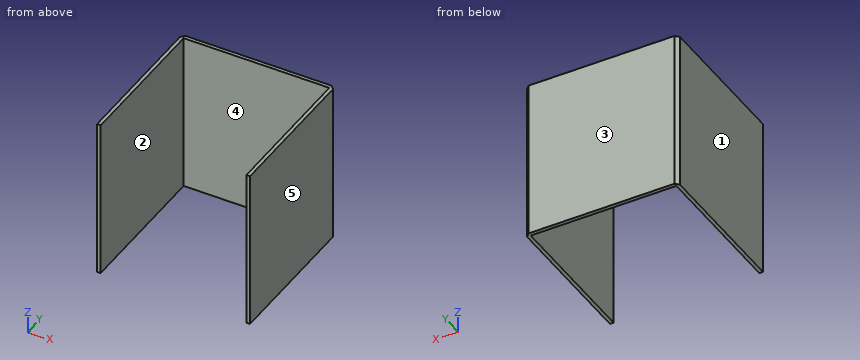
Autodesk Inventor part; units mm, degrees
ref_plane "YZ Plane" through (0, 0, 0) normal (1, 0, 0) x (0, 1, 0)
ref_plane "XZ Plane" through (0, 0, 0) normal (0, 1, 0) x (-1, 0, 0)
ref_plane "XY Plane" through (0, 0, 0) normal (0, 0, 1) x (1, 0, 0)
sketch "Sketch1" plane through (0, 0, 0) normal (0, 0, 1) x (1, 0, 0)
  line L0 (10, -10) -> (-10, -10)
  line L1 (-10, -10) -> (-10, 10)
  line L2 (-10, 10) -> (10, 10)
  line L3 (10, 10) -> (10, -10)
  line L4 (10, -10) -> (-10, 10) construction
  line L5 (-10, -10) -> (10, 10) construction
  line L6 (10.5, 10.5) -> (-10.5, 10.5)
  line L7 (-10.5, 10.5) -> (-10.5, -10.5)
  line L8 (-10.5, -10.5) -> (10.5, -10.5)
  line L9 (10.5, -10.5) -> (10.5, 10.5)
  line L10 (-10.5, -10) -> (10.5, -10)
  point P0 (0, 0)
  dimension "d0" = 20
  dimension "d1" = 20
  dimension "d2" = 0.5
extrude "Extrusion1" add sketch "Sketch1" along normal mid plane 22 contours L3 L2 L1 L10 L7 L6 L9
chamfer "Chamfer1" distance 0.5 angle 45 2 edges at (10.5, 10.5, 0) (-10.5, 10.5, 0)
properties part number "cover"
Can you work these out from the model? Positions are in its coordinate system, mm. Face numbers are marked on the shaded views. A direction names the side the tool comes from. Give positions to 0.01 mm unless a question says otherwise; leave off trailing zeros. Order: outer loops, then holes, each group sorted by start corner. A loop starts at its lowest first (then second) coordinate and runs counter-clockwise, first axis right, second up. Notation, with made-up numbers: M 34.25,84.5 L 64.25,84.5 A21 cw 64.25,107.5 Z; hole C 55.5,-5.75 d8. An arc over 180 degrees is marked long. Use one line per item in the form item = value.
Item 1: Will this pin go through, and if not, where does the flat tip stop? pin 1 Ø2 at (x, z) = (2.5, -5.5) entering from -Y.
Values follow:
pin_1 = 10
Item 2: If we section it at A-A, the plane y = -5: Write out the boundary of the cut face in (x, z), and give its area (3 significant figures).
Values follow:
outline = M -10.5,-11 L -10,-11 L -10,11 L -10.5,11 Z; M 10,-11 L 10.5,-11 L 10.5,11 L 10,11 Z
area = 22.0 mm^2
Item 3: If we section it at B-B, the plane z = -1.25: Write out the boundary of the cut face in (x, y).
Values follow:
outline = M -10.5,-10 L -10,-10 L -10,10 L 10,10 L 10,-10 L 10.5,-10 L 10.5,10 L 10,10.5 L -10,10.5 L -10.5,10 Z
Item 4: If we section it at C-C, the plane x = 7.25: Write out the boundary of the cut face in (y, z), and give its area (3 significant figures).
Values follow:
outline = M 10,-11 L 10.5,-11 L 10.5,11 L 10,11 Z
area = 11.0 mm^2
Item 5: Thinking about a two-plate mould opening in X: for the marked faces 1, 2 and 3, which applies, pulls with the +X half, pulls with the -X half, needs draft (parallel to the pull), parting line crosses it, or undercut?
Values follow:
face_1 = pulls with the -X half
face_2 = undercut
face_3 = needs draft
Item 6: If I drill on line 1 along X through (y, z) = (8, 7.5); line 2 along Y through (x, z) = (4.75, -8.5), over which ranges is the centre line in solid material (lowest first)? Write a range as [from, to].
Values follow:
line_1 = [-10.5, -10], [10, 10.5]
line_2 = [10, 10.5]
Item 7: For the marked faces 4 and 5, which set-ups out of +Z, -Z, +X, -X, +Y, -Y let a thin tool reach every point of the face, with its end or its side?
Values follow:
face_4 = +Z, -Z, -Y
face_5 = +Z, -Z, +X, +Y, -Y
